Design review of the part built by this model. Coordinates are the model's own, in mm. A direction names the side the tool comes from. Round coordinates to 2 decimals unless told otherwise and drop trailing zeros. Write each loop counter-clockwise with the first axis right and the second up, starting at its lowest first coordinate (ties: lowest second). Pieces come first, ordered by that corner, then holes. Notation, with made-up numbers: M 79.25,48.25 L 133.25,48.25 A26 cw 133.25,87.25 Z; hole C -29.75,-24 d3. An arc over 180 degrees is marked long. One line per question, with ' | ' between items. Start each with the question number.
Item 1: For L1, parallel to X at y = 0, z = 19.5; L2, parallel to Z at x = -30.5, y = 57; L3, parallel to X at y = 64, z = 9, list the stretches that pass through material, from the lowest coordinate up.
Item 2: Add section B-B, the plane z = 24.5. State the section outline as (x, y) points, and give its area (3 significant figures).
Item 3: Insertion check: pin 1 Ø1.5 at (x, z) = (-34.5, 25.5) entering from +Y; pin 2 Ø6 at (x, y) = (1.5, -2.5) entering from -Z; pin 3 Ø12 at (y, z) = (31, 31.5) entering from +X. Each pin has a flat end and moves straight along its axis. Give the tip position at first contact, or say it passes through.
Item 4: Draft analysis for pull direction Y (two halves, no side actions). For faces 1 (the face through (-53.436, 48.999, 18.734)), 2 (the face through (-15.066, 67.847, 18.241)), 3 (the face through (-37.4, -61.6, 13.2)), state which applies: released by +Y, released by -Y, zero draft, split by the parting line, or undercut.
Item 5: Machinability: for faces 4 (the face through (-1, -1, 37)), 5 (the face through (37.86, -61.58, 15.9)), 6 (the face through (-1, 1, 40)), which of the approach directions +Z, -Z, +X, -X, +Y, -Y give a long, thin tool a straight path to every point of the face, cutting with its end or side? Answer none if there is none.
Item 6: Add section C-C, the plane z = 15. State the section outline as (x, y) points, and give its area (3 significant figures).
Item 7: Add section A-A, the plane x = 0. State the section outline as (y, z) points.
```python
from build123d import *

# Parameters (mm, degrees)
F0_R          = 72.5
F1_DEPTH      = 40
F2_R          = 69.5
F3_DEPTH      = 37
F4_R          = 3
F5_DEPTH      = 72.501
F6_R          = 1.5
F7_DEPTH      = 72.5010001
F7_DEPTH_BACK = 72.5010001
F8_R          = 2


with BuildPart() as f1:
    # F0 (on Top) → F1 (new body)
    with BuildSketch(Plane.XY):
        Circle(F0_R)
    extrude(amount=F1_DEPTH)

    # F2 (on face) → F3 (cut)
    with BuildSketch(Plane(origin=(0, 0, 0), x_dir=(1, 0, 0), z_dir=(0, 0, -1))):
        Circle(F2_R)
    extrude(amount=-F3_DEPTH, mode=Mode.SUBTRACT)

    # F4 (on Front) → F5 (cut, through all)
    with BuildSketch(Plane.XZ):
        with Locations((35, 15)):
            Circle(F4_R)
        with Locations((-35, 15)):
            Circle(F4_R)
    extrude(amount=F5_DEPTH, mode=Mode.SUBTRACT)

    # F6 (on Right) → F7 (cut, two sides)
    with BuildSketch(Plane.YZ) as f7_sk:
        with Locations((0, 7)):
            Circle(F6_R)
    extrude(amount=-F7_DEPTH, mode=Mode.SUBTRACT)
    extrude(f7_sk.sketch, amount=F7_DEPTH_BACK, mode=Mode.SUBTRACT)

    # F8
    f8_edges = [f1.edges().sort_by_distance(p)[0] for p in [
        (-72.5, 0, 40),
    ]]
    fillet(f8_edges, radius=F8_R)


solid = f1.part
```
Computed values:
1) L1: x = -72.5 to -69.5, 69.5 to 72.5 | L2: z = 37 to 40 | L3: x = -34.06 to -27.1, 27.1 to 34.06
2) outline: C 0,0 d145; hole C 0,0 d139 | area: 1,340 mm^2
3) pin 1: stops at y = 64.17 | pin 2: stops at z = 37 | pin 3: stops at x = 68.05
4) face 1: split by the parting line | face 2: undercut | face 3: zero draft
5) face 4: -Z | face 5: -Y | face 6: +Z, +X, -X, +Y, -Y
6) outline: M -38,-61.74 L -38,-58.19 A69.5 cw long 38,-58.19 L 38,-61.74 A72.5 ccw long Z; M -32,-65.06 A72.5 ccw 32,-65.06 L 32,-61.69 A69.5 cw -32,-61.69 Z | area: 1,300 mm^2
7) outline: M -72.5,0 L -69.5,0 L -69.5,37 L 69.5,37 L 69.5,0 L 72.5,0 L 72.5,38 A2 ccw 70.5,40 L -70.5,40 A2 ccw -72.5,38 Z
